Check sheet for the modelled part. Datum: model origin and axes. Units: mm. A direction names the side the tool comes from. Coordinates: 2 decimals unless noted, no trailing zeros. Loops run counter-clockwise (first coordinate to the right, second up) from the corner with the lowest first, then second, coordinate; pieces in that order, holes last. Notation, with made-up numbers: M 5.25,58 L 56.25,58 A17 cw 56.25,74 Z; hole C 72.5,10.25 d5. An arc over 180 degrees is marked long. Use CSV: the item, a comma, the result in double quotes. Start each with the question number.
(1) Section check B-B on x = 7. Record the cut outline in (y, z), and give its area (3 significant figures).
(2) Draft check along Y on faces 1 (the cylindrical face through (2.72, 2.66, 2.52)), 2 (the flat face through (12, 10, 2)), 3 (the flat face through (16, 0, 1)). Enter one of: pulls with the +Y half, pulls with the -Y half, needs draft (parallel to the pull), parting line crosses it, or undercut.
(3) Set-up check for faces 4 (the cylindrical face through (2.72, -2.66, 2.52)), 5 (the flat face through (10, 7.2, 3.5)), 6 (the flat face through (10, 0, 2)): record each of +Z, -Z, +X, -X, +Y, -Y from which the full face is reachable in a straight line by a thin tool's end or side.
(4) Section check A-A on y = 0. Record the cut outline in (x, z).
(5) Go/stop test with flat-tipped pins: pin 1 Ø8 at (x, y) = (12, 2.5) entering from +Z; pin 2 Ø3 at (x, y) = (0.5, -1) entering from +Z; pin 3 Ø2 at (y, z) = (-3.5, 3) entering from -X; pin 4 Ø0.7 at (x, z) = (6.5, 1.5) entering from -Y. Record where each tip stops, or that it passes through.
(6) Scan lines: line 1 (X direction, y = -3, z = 1.45); line 2 (Z direction, x = 10.75, y = -5); line 3 (X direction, y = 2.75, z = 2.15). Record each from-to range of solid material in increasing order.
from build123d import *

# Parameters (mm, degrees)
SKETCH1_R           = 2.5
BOSS_EXTRUDE1_DEPTH = 4
SKETCH4_R           = 3.49
CUT_EXTRUDE1_DEPTH  = 3
SKETCH5_W           = 6
SKETCH5_H           = 20
CUT_EXTRUDE2_DEPTH  = 1
CUT_EXTRUDE3_REACH  = 21.287
FILLET1_R           = 0.5
FILLET2_R           = 1.5
FILLET3_R           = 0.5


with BuildPart() as part:
    # Sketch1 → Boss-Extrude1 (new body)
    with BuildSketch(Plane.XY):
        with BuildLine():
            Line((-2.374946989, 4.399957591), (8, 10))
            Line((8, 10), (16, 10))
            Line((16, 10), (16, -10))
            Line((16, -10), (8, -10))
            Line((8, -10), (-2.374946989, -4.399957591))
            ThreePointArc((-2.374946989, -4.399957591), (-5, 0), (-2.374946989, 4.399957591))
        make_face()
        Circle(SKETCH1_R, mode=Mode.SUBTRACT)
    extrude(amount=BOSS_EXTRUDE1_DEPTH)

    # Sketch4 → Cut-Extrude1 (cut)
    with BuildSketch(Plane.XY.offset(4)):
        Circle(SKETCH4_R)
    extrude(amount=-CUT_EXTRUDE1_DEPTH, mode=Mode.SUBTRACT)

    # Sketch5 → Cut-Extrude2 (cut)
    with BuildSketch(Plane.XY.offset(4)):
        with Locations((13, 0)):
            Rectangle(SKETCH5_W, SKETCH5_H)
    extrude(amount=-CUT_EXTRUDE2_DEPTH, mode=Mode.SUBTRACT)

    # Sketch6 → Cut-Extrude3 (cut, up to next)
    with BuildSketch(Plane.XY.offset(4), mode=Mode.PRIVATE) as cut_extrude3_sk1:
        Polygon((3, 5.150585296), (5.5, 6.5), (8, 6.5), (8, 4.5), (10, 4.5), (10, -4.5), (8, -4.5), (8, -6.5), (5.5, -6.5), (3, -5.150585296), align=None)
    cut_extrude3_tool1 = extrude(cut_extrude3_sk1.sketch, amount=-CUT_EXTRUDE3_REACH, mode=Mode.PRIVATE) & part.part
    add(cut_extrude3_tool1.solids().sort_by_distance((6.361806, 0, 4))[0], mode=Mode.SUBTRACT)

    # Fillet1
    fillet1_edges = [part.edges().sort_by_distance(p)[0] for p in [
        (3, -1.783283488, 2.5),
        (3, 1.783283488, 2.5),
    ]]
    fillet(fillet1_edges, radius=FILLET1_R)

    # Fillet2
    fillet2_edges = [part.edges().sort_by_distance(p)[0] for p in [
        (10, 4.5, 1.5),
        (3, -5.150585296, 2),
        (3, 5.150585296, 2),
        (5.5, 6.5, 2),
        (8, 6.5, 2),
        (10, -4.5, 1.5),
        (8, -6.5, 2),
        (5.5, -6.5, 2),
    ]]
    fillet(fillet2_edges, radius=FILLET2_R)

    # Fillet3
    fillet3_edges = [part.edges().sort_by_distance(p)[0] for p in [
        (8, -4.5, 2),
        (8, 4.5, 2),
    ]]
    fillet(fillet3_edges, radius=FILLET3_R - 0.0001)  # a hair under: the kernel refuses the full size


solid = part.part
Outcome:
1,outline,"M -9.46,0 L -6.41,0 L -6.41,4 L -9.46,4 Z; M 6.41,0 L 9.46,0 L 9.46,4 L 6.41,4 Z"
1,area,"24.4 mm²"
2,face 1,"undercut"
2,face 2,"pulls with the +Y half"
2,face 3,"needs draft"
3,face 4,"+Z"
3,face 5,"+Z, +X, +Y, -Y"
3,face 6,"+Z, -Z"
4,outline,"M -5,0 L -2.5,0 L -2.5,1 L -3.49,1 L -3.49,4 L -5,4 Z; M 2.5,0 L 3,0 L 3,1 L 2.5,1 Z; M 10,0 L 16,0 L 16,3 L 10,3 Z"
5,pin 1,"stops at z = 4"
5,pin 2,"stops at z = 1"
5,pin 3,"stops at x = -4.33"
5,pin 4,"stops at y = -9.38"
6,line 1,"x = -4 to -1.78, 1.78 to 2.99, 10 to 16"
6,line 2,"z = 0 to 3"
6,line 3,"x = -4.18 to -2.15, 2.15 to 2.85, 10 to 16"
